```python
from build123d import *

# Parameters (mm, degrees)
SKETCH4_R            = 6
BOSS_EXTRUDE2_DEPTH  = 12
BOSS_EXTRUDE3_DEPTH  = 30
SKETCH16_R           = 2
BOSS_EXTRUDE9_DEPTH  = 8.5
SKETCH17_R           = 2
BOSS_EXTRUDE10_DEPTH = 8.5
BOSS_EXTRUDE11_DEPTH = 6
SKETCH20_W           = 15
SKETCH20_H           = 6
BOSS_EXTRUDE12_DEPTH = 6
SKETCH22_R           = 3
BOSS_EXTRUDE13_DEPTH = 1
SKETCH23_R           = 3
BOSS_EXTRUDE14_DEPTH = 1
SKETCH27_R           = 1.25
CUT_EXTRUDE4_DEPTH   = 16
SKETCH28_R           = 1.5
CUT_EXTRUDE5_DEPTH   = 17


with BuildPart() as part:
    # Sketch4 → Boss-Extrude2 (new body)
    with BuildSketch(Plane(origin=(0, 0, 0), x_dir=(1, 0, 0), z_dir=(0, 1, 0))):
        with BuildLine():
            Line((0, 28.214565602), (0, -28.214565602))
            Line((0, -28.214565602), (114.556109318, -28.214565602))
            Line((114.556109318, -28.214565602), (125.637290842, -9.021396193))
            Line((125.637290842, -9.021396193), (170.11344646, -9.021396193))
            ThreePointArc((170.11344646, -9.021396193), (191.265868706, 0), (170.11344646, 9.021396193))
            Line((170.11344646, 9.021396193), (125.637290842, 9.021396193))
            Line((125.637290842, 9.021396193), (114.556109318, 28.214565602))
            Line((114.556109318, 28.214565602), (0, 28.214565602))
        make_face()
        with Locations((178.765868706, 0)):
            Circle(SKETCH4_R, mode=Mode.SUBTRACT)
    extrude(amount=BOSS_EXTRUDE2_DEPTH)

    # Sketch6 → Boss-Extrude3 (add)
    with BuildSketch(Plane(origin=(0, 12, 0), x_dir=(1, 0, 0), z_dir=(0, 1, 0))):
        Polygon((0, 0), (0, 28.214565602), (114.556109318, 28.214565602), (125.637290842, 9.021396193), (130.845796363, 0), (114.556109318, -28.214565602), (0, -28.214565602), align=None)
    extrude(amount=BOSS_EXTRUDE3_DEPTH)

    # Mirror5: part across plane


with BuildPart() as part_1:
    add(part.part)
    add(part.part.mirror(Plane(origin=(0, 42, 0), x_dir=(0, 0, 1), z_dir=(0, -1, 0))))

    # Sketch16 → Boss-Extrude9 (add)
    with BuildSketch(Plane(origin=(98.134347272, 0, -56.657891814), x_dir=(-0.5, 0, -0.866025404), z_dir=(0.866025404, 0, -0.5))):
        with Locations((-52.407887359, 29)):
            Circle(SKETCH16_R)
    extrude(amount=BOSS_EXTRUDE9_DEPTH)

    # Sketch17 → Boss-Extrude10 (add)
    with BuildSketch(Plane(origin=(98.134347272, 0, 56.657891814), x_dir=(0.5, 0, -0.866025404), z_dir=(0.866025404, 0, 0.5))):
        with Locations((52.407887359, 35)):
            Circle(SKETCH17_R)
    extrude(amount=BOSS_EXTRUDE10_DEPTH)

    # Sketch18 → Boss-Extrude11 (add)
    with BuildSketch(Plane(origin=(98.134347272, 0, -56.657891814), x_dir=(-0.5, 0, -0.866025404), z_dir=(0.866025404, 0, -0.5))):
        Polygon((-32.843524091, 59), (-32.843524091, 56.190441435), (-45.940020371, 56.190441435), (-45.940020371, 62.190441435), (-32.843524091, 62.190441435), align=None)
    extrude(amount=BOSS_EXTRUDE11_DEPTH)

    # Sketch20 → Boss-Extrude12 (add)
    with BuildSketch(Plane(origin=(98.134347272, 0, 56.657891814), x_dir=(0.5, 0, -0.866025404), z_dir=(0.866025404, 0, 0.5))):
        with Locations((40.343524091, 65)):
            Rectangle(SKETCH20_W, SKETCH20_H)
    extrude(amount=BOSS_EXTRUDE12_DEPTH)

    # Sketch22 → Boss-Extrude13 (add)
    with BuildSketch(Plane(origin=(105.495563204, 0, -60.907891814), x_dir=(-0.5, 0, -0.866025404), z_dir=(0.866025404, 0, -0.5))):
        with Locations((-52.407887359, 29)):
            Circle(SKETCH22_R)
    extrude(amount=-BOSS_EXTRUDE13_DEPTH)

    # Sketch23 → Boss-Extrude14 (add)
    with BuildSketch(Plane(origin=(105.495563204, 0, 60.907891814), x_dir=(0.5, 0, -0.866025404), z_dir=(0.866025404, 0, 0.5))):
        with Locations((52.407887359, 35)):
            Circle(SKETCH23_R)
    extrude(amount=-BOSS_EXTRUDE14_DEPTH)

    # Sketch27 → Cut-Extrude4 (cut)
    with BuildSketch(Plane(origin=(16.421762045, 0, 28.443326212), x_dir=(-0.866025404, 0, 0.5), z_dir=(-0.5, 0, -0.866025404))):
        with Locations((-117.315783629, 59.190441435)):
            Circle(SKETCH27_R)
    extrude(amount=-CUT_EXTRUDE4_DEPTH, mode=Mode.SUBTRACT)

    # Sketch28 → Cut-Extrude5 (cut)
    with BuildSketch(Plane(origin=(23.921762045, 0, -41.433707269), x_dir=(-0.866025404, 0, -0.5), z_dir=(0.5, 0, -0.866025404))):
        with Locations((-116.315783629, 65)):
            Circle(SKETCH28_R)
    extrude(amount=-CUT_EXTRUDE5_DEPTH, mode=Mode.SUBTRACT)


solid = part_1.part
```
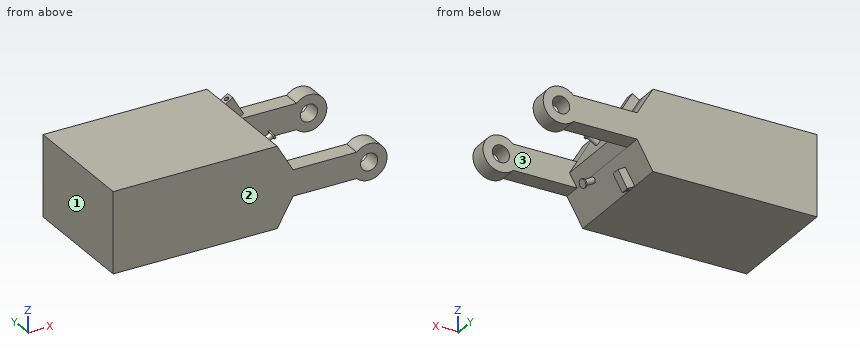
Input: part model. Units: mm. Frame: model coordinates. Face numbers are marked on the shaded views. Give positions to 0.01 mm unless a question says otherwise; leave off trailing zeros. Order: outer loops, then holes, each group sorted by start corner. A loop starts at its lowest first (then second) coordinate and runs counter-clockwise, first axis right, second up. Notation, with made-up numbers: (-13, 9.5) - (22, 9.5) arc R25 ccw to (22, 30.5) - close; hole circle Ø8 at (61.5, 34). An arc over 180 degrees is marked (long way). One line per item, written item: value.
1. Cut plane A-A, the plane x = 175. Output: boundary loops of the cut face in (y, z), and give its area (3 significant figures).
Determined:
outline: (0, -11.92) - (12, -11.92) - (12, -4.67) - (0, -4.67) - close; (0, 4.67) - (12, 4.67) - (12, 11.92) - (0, 11.92) - close; (72, -11.92) - (84, -11.92) - (84, -4.67) - (72, -4.67) - close; (72, 4.67) - (84, 4.67) - (84, 11.92) - (72, 11.92) - close
area: 348 mm2
2. Pin query (flat end, axial travel): pin 1 Ø6.5 at (x, z) = (123, 27) entering from +Y; pin 2 Ø6 at (x, z) = (123, -27.5) entering from -Y; pin 3 Ø3 at (x, y) = (71, 62) entering from -Z. Return the tip coordinate at first contact, or that it passes through.
Determined:
pin 1: y = 68
pin 2: y = 56.19
pin 3: z = -28.21
3. Draft query along Y for the marked faces 1, 2 and 3. Return one class per face: released by +Y, released by -Y, zero draft, split by the parting line, or undercut.
Determined:
face 1: zero draft
face 2: released by -Y
face 3: undercut
4. Line query: probe 1 along Y at (x, z) = (155, 0); probe 2 along Z at (x, y) = (74.5, 40.5); probe 3 along X at (y, z) = (44, -13). Output: solid intervals per line, ascending.
Determined:
probe 1: 0 to 12, 72 to 84
probe 2: -28.21 to 28.21
probe 3: 0 to 123.34
5. Cut plane B-B, the plane y = 52. Output: boundary loops of the cut face in (x, z), and give its area (3 significant figures).
Determined:
outline: (0, -28.21) - (114.56, -28.21) - (130.85, 0) - (114.56, 28.21) - (0, 28.21) - close
area: 6,920 mm2
6. Cut plane C-C, the plane x = 77.5. Output: boundary loops of the cut face in (y, z).
Determined:
outline: (0, -28.21) - (84, -28.21) - (84, 28.21) - (0, 28.21) - close
